from build123d import *

# Parameters (mm, degrees)
SKETCH_R      = 74
SKETCH_R_2    = 71
PAD_DEPTH     = 13.5
SKETCH001_R   = 74
SKETCH001_R_2 = 67.5
PAD001_DEPTH  = 3
SKETCH002_W   = 30
SKETCH002_H   = 30
PAD002_DEPTH  = 5
SKETCH003_R   = 3
POCKET_DEPTH  = 5
CHAMFER_SIZE2 = 4
CHAMFER_SIZE  = 11
FILLET_R      = 13


with BuildPart() as part:
    # Sketch → Pad (new body)
    with BuildSketch(Plane.XY):
        Circle(SKETCH_R)
        Circle(SKETCH_R_2, mode=Mode.SUBTRACT)
    extrude(amount=PAD_DEPTH)

    # Sketch001 (on Face4 of Pad) → Pad001 (join)
    with BuildSketch(Plane.XY.offset(13.5)):
        Circle(SKETCH001_R)
        Circle(SKETCH001_R_2, mode=Mode.SUBTRACT)
    extrude(amount=PAD001_DEPTH)

    # Sketch002 (on Face1 of Pad001) → Pad002 (join)
    with BuildSketch(Plane(origin=(0, 0, 0), x_dir=(1, 0, 0), z_dir=(0, 0, -1))):
        with Locations((87, 0)):
            Rectangle(SKETCH002_W, SKETCH002_H)
        with Locations((0, 87)):
            Rectangle(SKETCH002_W, SKETCH002_H)
        with Locations((-87, 0)):
            Rectangle(SKETCH002_W, SKETCH002_H)
        with Locations((0, -87)):
            Rectangle(SKETCH002_W, SKETCH002_H)
    extrude(amount=-PAD002_DEPTH)

    # Sketch003 (on Face10 of Pad002) → Pocket (cut)
    with BuildSketch(Plane.XY.offset(5)):
        with Locations((86.25, 0)):
            Circle(SKETCH003_R)
        with Locations((0, 86.25)):
            Circle(SKETCH003_R)
        with Locations((-86.25, 0)):
            Circle(SKETCH003_R)
        with Locations((0, -86.25)):
            Circle(SKETCH003_R)
    extrude(amount=-POCKET_DEPTH, mode=Mode.SUBTRACT)

    # Chamfer
    chamfer_edges = [part.edges().sort_by_distance(p)[0] for p in [
        (0, 74, 5),
        (73.614944, 7.53923, 5),
        (0, -74, 5),
        (-74, 0, 5),
    ]]
    chamfer_side = part.faces().sort_by_distance((-74, 0, 8.25))[0]
    chamfer(chamfer_edges, length=CHAMFER_SIZE, length2=CHAMFER_SIZE2, reference=chamfer_side)

    # Fillet
    fillet_edges = [part.edges().sort_by_distance(p)[0] for p in [
        (15, 102, 2.5),
        (-15, 102, 2.5),
        (102, 15, 2.5),
        (102, -15, 2.5),
        (15, -102, 2.5),
        (-15, -102, 2.5),
        (-102, -15, 2.5),
        (-102, 15, 2.5),
    ]]
    fillet(fillet_edges, radius=FILLET_R)


solid = part.part
Geometry: final body of the model. Coordinates: model frame, mm. A direction names the side the tool comes from. Coordinates: 2 decimals unless noted, no trailing zeros. Order: outer loops, then holes, each group sorted by start corner. A loop starts at its lowest first (then second) coordinate and runs counter-clockwise, first axis right, second up.
1) Section C-C (x = -47). Return loops of the section in (y, z), then the cut area to 3 significant figures.
Result sheet:
outline: (-57.16, 0) - (-53.22, 0) - (-53.22, 13.5) - (-48.45, 13.5) - (-48.45, 16.5) - (-57.16, 16.5) - close; (48.45, 13.5) - (53.22, 13.5) - (53.22, 0) - (57.16, 0) - (57.16, 16.5) - (48.45, 16.5) - close
area: 159 mm2
2) First-contact query: P1, Ø2, axis at x = 14.5, z = 8, coming from the +Y side; P2, Ø5.5, axis at x = 0, y = -86.25, coming from the -Z side; P3, Ø8, axis at x = -81.5, z = 8.5, coming from the +Y side; P4, Ø20.5, axis at x = -5.5, y = 95.5, coming from the +Z side. Flat tips, straight axial feed; report the tip coordinate or a pass-through.
Result sheet:
P1: stops at y = 75.95
P2: passes through
P3: stops at y = 15
P4: stops at z = 5
3) Section D-D (y = -19). Return loops of the section in (x, z), then the cut area to 3 significant figures.
Result sheet:
outline: (-71.52, 0) - (-68.41, 0) - (-68.41, 13.5) - (-64.77, 13.5) - (-64.77, 16.5) - (-71.52, 16.5) - close; (64.77, 13.5) - (68.41, 13.5) - (68.41, 0) - (71.52, 0) - (71.52, 16.5) - (64.77, 16.5) - close
area: 124 mm2
4) Draft query along Y for faces 6 (the cylindrical face through (34.15, -65.65, 8.13)), 7 (the cylindrical face through (-98.091, 11.293, 2.535)), 8 (the cylindrical face through (83.253, 0.132, 2.535)). Return one class per face: released by +Y, released by -Y, zero draft, split by the parting line, or undercut.
Result sheet:
face 6: split by the parting line
face 7: released by +Y
face 8: undercut
5) Section A-A (y = -86.25). Return loops of the section in (x, z), then the cut area to 3 significant figures.
Result sheet:
outline: (-15, 0) - (-3, 0) - (-3, 5) - (-15, 5) - close; (3, 0) - (15, 0) - (15, 5) - (3, 5) - close
area: 120 mm2
6) Ray query, probe 1 along Y at (x, z) = (0, 3.4); probe 2 along Y at (x, z) = (-86.25, 2.85); probe 3 along X at (y, z) = (-73.5, 7.25). Return the intervals inside material, ascending.
Result sheet:
probe 1: y = -102 to -89.25, -83.25 to -71, 71 to 83.25, 89.25 to 102
probe 2: y = -15 to -3, 3 to 15
probe 3: x = -15 to 15
7) Set-up query: faces 1 (the cylindrical face through (-15.39, -69.31, 6.66)), 2 (the flat face through (-15, -79, 4)), 3 (the flat face through (15, 79, 4)), 4 (the flat face through (79, -15, 4)), 5 (the cylindrical face through (-11.091, 98.293, 2.535)). Return all of +Z, -Z, +X, -X, +Y, -Y with unobstructed straight access to the full face (end or side cutting, diameter ignored); none if empty.
Result sheet:
face 1: -Z
face 2: +Z, -Z, -X, -Y
face 3: +Z, -Z, +X, +Y
face 4: +Z, -Z, +X, -Y
face 5: +Z, -Z, -X, +Y
